Check sheet for the drawn part. Datum: minimum x, y, z corner. Units: mm. Round coordinates to 2 decimals unless told otherwise and drop trailing zeros. Write each loop counter-clockwise with the first axis right and the second up, starting at its lowest first coordinate (ties: lowest second). Pieces come first, ordered by that corner, then holes. Notation, with made-up numbers: (-31.5, -29) -> (-26.5, -29) arc R25 ccw to (-26.5, -10) -> close; hole circle Ø9 at (36, -24). An arc over 180 degrees is marked (long way). One line per item, written item: value.
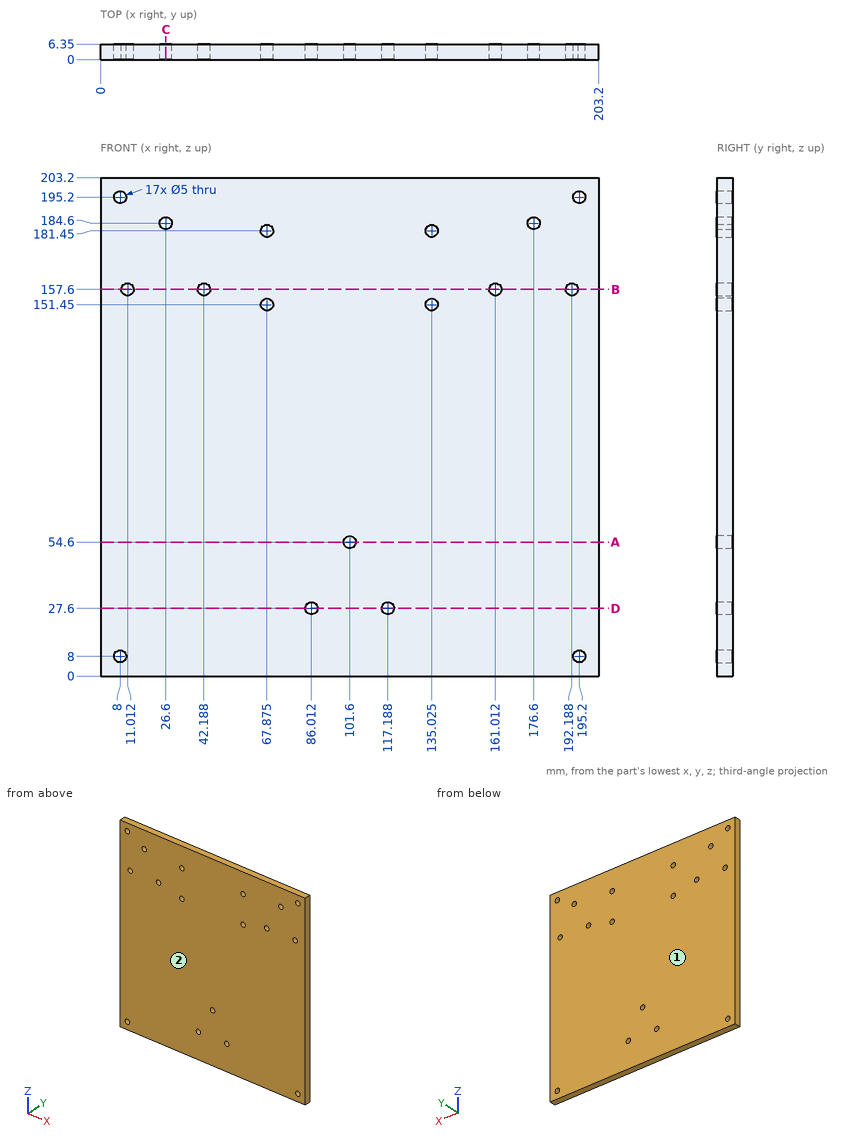
Item 1: Sectioned sample at B-B on z = 157.6. Enter the section's corners in (x, y), and give its area (3 significant figures).
Answer:
outline: (0, 0) -> (8.51, 0) -> (8.51, 6.35) -> (0, 6.35) -> close; (13.51, 0) -> (39.69, 0) -> (39.69, 6.35) -> (13.51, 6.35) -> close; (44.69, 0) -> (158.51, 0) -> (158.51, 6.35) -> (44.69, 6.35) -> close; (163.51, 0) -> (189.69, 0) -> (189.69, 6.35) -> (163.51, 6.35) -> close; (194.69, 0) -> (203.2, 0) -> (203.2, 6.35) -> (194.69, 6.35) -> close
area: 1,160 mm^2
Item 2: Sectioned sample at C-C on x = 26.6. Enter the section's corners in (y, z).
Answer:
outline: (0, 0) -> (6.35, 0) -> (6.35, 182.1) -> (0, 182.1) -> close; (0, 187.1) -> (6.35, 187.1) -> (6.35, 203.2) -> (0, 203.2) -> close
Item 3: Mould release check, pull along Y, two halves, no side actions. Record for the marked faces 1 and 2: pulls with the +Y half, pulls with the -Y half, needs draft (parallel to the pull), parting line crosses it, or undercut.
Answer:
face 1: pulls with the +Y half
face 2: pulls with the -Y half
Item 4: Sectioned sample at A-A on z = 54.6. Enter the section's corners in (x, y), and give its area (3 significant figures).
Answer:
outline: (0, 0) -> (99.1, 0) -> (99.1, 6.35) -> (0, 6.35) -> close; (104.1, 0) -> (203.2, 0) -> (203.2, 6.35) -> (104.1, 6.35) -> close
area: 1,260 mm^2
Item 5: Thickness scan on line 1 (X direction, y = 4.25, z = 27.6); line 2 (Z direction, x = 135, y = 4.5); line 3 (X direction, y = 2.25, z = 181.45) (1 decimal). Record the ranges inside material, lowest first.
Answer:
line 1: x = 0 to 83.51, 88.51 to 114.69, 119.69 to 203.2
line 2: z = 0 to 148.95, 153.95 to 178.95, 183.95 to 203.2
line 3: x = 0 to 65.4, 70.4 to 132.5, 137.5 to 203.2
Item 6: Sectioned sample at D-D on z = 27.6. Enter the section's corners in (x, y), and give its area (3 significant figures).
Answer:
outline: (0, 0) -> (83.51, 0) -> (83.51, 6.35) -> (0, 6.35) -> close; (88.51, 0) -> (114.69, 0) -> (114.69, 6.35) -> (88.51, 6.35) -> close; (119.69, 0) -> (203.2, 0) -> (203.2, 6.35) -> (119.69, 6.35) -> close
area: 1,230 mm^2
